The model under review builds one solid part; all positions refer to its coordinate system, in mm. A direction names the side the tool comes from. Give positions to 0.01 mm unless a question says otherwise; leave off trailing zeros. Loops run counter-clockwise (first coordinate to the right, second up) from the corner with the lowest first, then second, coordinate; pieces in that order, holes last. Notation, with made-up numbers: M 36,-31.75 L 70,-31.75 A22 cw 70,-21.75 Z; hole C 53,16 d3. An arc over 180 degrees is marked long. One line per item, written item: value. Start each with the question number.
Q1. For pin 1 (4 mm diameter, centred on x = 10, z = 40, fed in from -Y), flat-tipped, find the tip position at first contact; note if it passes through.
Q2. For faces 4 (the face through (10, 18, 197)), 5 (the face through (10, 20, 197)), list the 3-axis set-ups (+Z, -Z, +X, -X, +Y, -Y) from which the entire face can be reached by the end or side of a thin tool; tool diameter is ignored.
Q3. Mouldability with a two-part tool opening along X and no side actions: class faces 1 (the face through (1, 10, 0)), 2 (the face through (20, 10, 197)), 3 (the face through (2, 10, 197)) as released by +X, released by -X, zero draft, split by the parting line, or undercut.
Q4. To check wall thickness, follow line 1 along X through (y, z) = (15, 37); line 2 along X through (y, z) = (18.55, 320). State the ranges of each line that lie inside material, in increasing order. Write a range as from..to.
Q5. We need section B-B on z = 285. Write out the cut boundary in (x, y).
Q6. We need section A-A on x = 15. Write out the cut boundary in (y, z), plus the area to 3 significant figures.
```python
from build123d import *

# Parameters (mm, degrees)
SKETCH_1_W          = 20
SKETCH_1_H          = 20
SKETCH_1_W_2        = 16
SKETCH_1_H_2        = 16
EXTRUDE_1_DEPTH     = 400
SKETCH_9_R          = 1.5
CUT_EXTRUDE_6_DEPTH = 401.998753115


with BuildPart() as part:
    # 草图1 → 凸台-拉伸1 (new body)
    with BuildSketch(Plane.XY):
        with Locations((10, 10)):
            Rectangle(SKETCH_1_W, SKETCH_1_H)
        with Locations((10, 10)):
            Rectangle(SKETCH_1_W_2, SKETCH_1_H_2, mode=Mode.SUBTRACT)
    extrude(amount=EXTRUDE_1_DEPTH)

    # 草图9 → 切除-拉伸6 (cut, through all)
    with BuildSketch(Plane(origin=(0, 20, 0), x_dir=(1, 0, 0), z_dir=(0, 1, 0))):
        with Locations(Location((10, -390, 0), (0, 0, 270))):
            Circle(SKETCH_9_R)
        with Locations(Location((10, -380, 0), (0, 0, 270))):
            Circle(SKETCH_9_R)
        with Locations(Location((10, -370, 0), (0, 0, 270))):
            Circle(SKETCH_9_R)
        with Locations(Location((10, -360, 0), (0, 0, 270))):
            Circle(SKETCH_9_R)
        with Locations(Location((10, -350, 0), (0, 0, 270))):
            Circle(SKETCH_9_R)
        with Locations(Location((10, -340, 0), (0, 0, 270))):
            Circle(SKETCH_9_R)
        with Locations(Location((10, -330, 0), (0, 0, 270))):
            Circle(SKETCH_9_R)
        with Locations(Location((10, -320, 0), (0, 0, 270))):
            Circle(SKETCH_9_R)
        with Locations(Location((10, -310, 0), (0, 0, 270))):
            Circle(SKETCH_9_R)
        with Locations(Location((10, -300, 0), (0, 0, 270))):
            Circle(SKETCH_9_R)
        with Locations(Location((10, -290, 0), (0, 0, 270))):
            Circle(SKETCH_9_R)
        with Locations(Location((10, -280, 0), (0, 0, 270))):
            Circle(SKETCH_9_R)
        with Locations(Location((10, -270, 0), (0, 0, 270))):
            Circle(SKETCH_9_R)
        with Locations(Location((10, -260, 0), (0, 0, 270))):
            Circle(SKETCH_9_R)
        with Locations(Location((10, -250, 0), (0, 0, 270))):
            Circle(SKETCH_9_R)
        with Locations(Location((10, -240, 0), (0, 0, 270))):
            Circle(SKETCH_9_R)
        with Locations(Location((10, -230, 0), (0, 0, 270))):
            Circle(SKETCH_9_R)
        with Locations(Location((10, -220, 0), (0, 0, 270))):
            Circle(SKETCH_9_R)
        with Locations(Location((10, -210, 0), (0, 0, 270))):
            Circle(SKETCH_9_R)
        with Locations(Location((10, -200, 0), (0, 0, 270))):
            Circle(SKETCH_9_R)
        with Locations(Location((10, -190, 0), (0, 0, 270))):
            Circle(SKETCH_9_R)
        with Locations(Location((10, -180, 0), (0, 0, 270))):
            Circle(SKETCH_9_R)
        with Locations(Location((10, -170, 0), (0, 0, 270))):
            Circle(SKETCH_9_R)
        with Locations(Location((10, -160, 0), (0, 0, 270))):
            Circle(SKETCH_9_R)
        with Locations(Location((10, -150, 0), (0, 0, 270))):
            Circle(SKETCH_9_R)
        with Locations(Location((10, -140, 0), (0, 0, 270))):
            Circle(SKETCH_9_R)
        with Locations(Location((10, -130, 0), (0, 0, 270))):
            Circle(SKETCH_9_R)
        with Locations(Location((10, -120, 0), (0, 0, 270))):
            Circle(SKETCH_9_R)
        with Locations(Location((10, -110, 0), (0, 0, 270))):
            Circle(SKETCH_9_R)
        with Locations(Location((10, -100, 0), (0, 0, 270))):
            Circle(SKETCH_9_R)
        with Locations(Location((10, -90, 0), (0, 0, 270))):
            Circle(SKETCH_9_R)
        with Locations(Location((10, -80, 0), (0, 0, 270))):
            Circle(SKETCH_9_R)
        with Locations(Location((10, -70, 0), (0, 0, 270))):
            Circle(SKETCH_9_R)
        with Locations(Location((10, -60, 0), (0, 0, 270))):
            Circle(SKETCH_9_R)
        with Locations(Location((10, -50, 0), (0, 0, 270))):
            Circle(SKETCH_9_R)
        with Locations(Location((10, -40, 0), (0, 0, 270))):
            Circle(SKETCH_9_R)
        with Locations(Location((10, -30, 0), (0, 0, 270))):
            Circle(SKETCH_9_R)
        with Locations(Location((10, -20, 0), (0, 0, 270))):
            Circle(SKETCH_9_R)
        with Locations(Location((10, -10, 0), (0, 0, 270))):
            Circle(SKETCH_9_R)
    extrude(amount=-CUT_EXTRUDE_6_DEPTH, mode=Mode.SUBTRACT)


solid = part.part
```
Solved:
1. pin 1: y = 0
2. face 4: +Z, -Z
2. face 5: +Z, -Z, +X, -X, +Y
3. face 1: zero draft
3. face 2: released by +X
3. face 3: undercut
4. line 1: 0..2, 18..20
4. line 2: 0..8.5, 11.5..20
5. outline: M 0,0 L 20,0 L 20,20 L 0,20 Z; hole M 2,2 L 18,2 L 18,18 L 2,18 Z
6. outline: M 0,0 L 2,0 L 2,400 L 0,400 Z; M 18,0 L 20,0 L 20,400 L 18,400 Z
6. area: 1,600 mm2
